Design review of the part built by this model. Coordinates are the model's own, in mm. Give positions to 0.01 mm unless a question says otherwise; leave off trailing zeros. Write each loop counter-clockwise with the first axis right and the second up, starting at its lowest first coordinate (ties: lowest second). Pieces come first, ordered by that corner, then holes. Notation, with made-up numbers: (78, 70.5) -> (128, 70.5) arc R19 cw to (128, 93.5) -> close; hole circle Ø8 at (86, -17.75). An arc over 180 degrees is marked (long way). Answer as a JSON object with one key per item and string values.
```python
from build123d import *

# Parameters (mm, degrees)
SM_GUIDE_DEPTH  = 416
SK_HOLES_R      = 2.15
CUT_HOLES_DEPTH = 1.5


# Sheet-metal steps are written as plain solids
with BuildPart() as part:
    # SK_Guide → SM_Guide (new body)
    with BuildSketch(Plane.XY.offset(-208)):
        with BuildLine():
            Line((48, 0), (63.5, 0))
            ThreePointArc((63.5, 0), (64.560660172, 0.439339828), (65, 1.5))
            Line((65, 1.5), (65, 20))
            Line((65, 20), (66.5, 20))
            Line((66.5, 20), (66.5, 1.5))
            ThreePointArc((66.5, 1.5), (65.621320344, -0.621320344), (63.5, -1.5))
            Line((63.5, -1.5), (48, -1.5))
            Line((48, -1.5), (48, 0))
        make_face()
    extrude(amount=SM_GUIDE_DEPTH)

    # SK_Holes → CUT_Holes (cut)
    with BuildSketch(Plane(origin=(0, 0, 0), x_dir=(1, 0, 0), z_dir=(0, 1, 0))):
        with Locations(Location((56, -198, 0), (0, 0, 270))):
            Circle(SK_HOLES_R)
        with Locations(Location((56, 198, 0), (0, 0, 270))):
            Circle(SK_HOLES_R)
    extrude(amount=-CUT_HOLES_DEPTH, mode=Mode.SUBTRACT)


solid = part.part
```
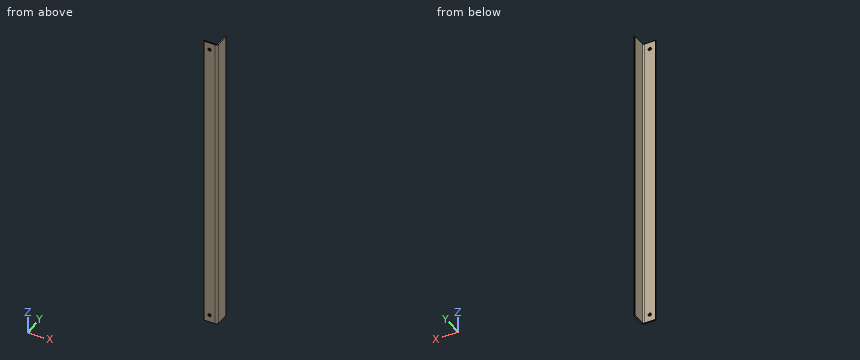
(1) For line 1 along X through (y, z) = (3.5, 106.5); line 2 along Y through (x, z) = (62.5, -104); line 3 along X through (y, z) = (-0.75, 198), list the stretches that pass through material, from the lowest coordinate up.
Here are the results:
{"line 1": "x = 65 to 66.5", "line 2": "y = -1.5 to 0", "line 3": "x = 48 to 53.85, 58.15 to 65.48"}
(2) Clearance check with flat-ended pins moving along their axes: pin 1 (2 mm diameter, centred on y = 13.5, z = -70.5, fed in from -X); pin 2 (10 mm diameter, centred on x = 50.5, z = 72, fed in from +Y); pin 3 (3.5 mm diameter, centred on x = 56, z = -198, fed in from -Y). State where each tip first meets the part, or that it passes through.
Here are the results:
{"pin 1": "stops at x = 65", "pin 2": "stops at y = 0", "pin 3": "passes through"}
(3) We need section B-B, the plane y = 8.5. State the section outline as (x, z) points.
Here are the results:
{"outline": "(65, -208) -> (66.5, -208) -> (66.5, 208) -> (65, 208) -> close"}
(4) We need section A-A, the plane z = -21. State the section outline as (x, y) points, then the cut area to 3 significant figures.
Here are the results:
{"outline": "(48, -1.5) -> (63.5, -1.5) arc R3 ccw to (66.5, 1.5) -> (66.5, 20) -> (65, 20) -> (65, 1.5) arc R1.5 cw to (63.5, 0) -> (48, 0) -> close", "area": "56.3 mm²"}
